```python
from build123d import *

# Parameters (mm, degrees)
F0_R      = 7.5
F1_DEPTH  = 5
F1_FACE_R = 7.5
F2_DEPTH  = 10
F2_TAPER  = 20


with BuildPart() as f1:
    # F0 (on Top) → F1 (new body)
    with BuildSketch(Plane.XY):
        Circle(F0_R)
    extrude(amount=F1_DEPTH)

    # F1_face (on face) → F2 (join)
    with BuildSketch(Plane.XY.offset(5)):
        Circle(F1_FACE_R)
    extrude(amount=F2_DEPTH, taper=F2_TAPER)

    # F3 (on Front) → F4 (revolve)
    with BuildSketch(Plane.XZ):
        with BuildLine():
            Line((0, 23), (0, 10))
            ThreePointArc((0, 10), (6.5, 16.5), (0, 23))
        make_face()
    revolve(axis=Axis((0, 0, 16.5), (0, 0, 1)))


solid = f1.part
```
Can you work these out from the model? Positions are in its coordinate system, mm. Give positions to 0.01 mm unless a question says otherwise; leave off trailing zeros. Loops run counter-clockwise (first coordinate to the right, second up) from the corner with the lowest first, then second, coordinate; pieces in that order, holes last. Notation, with made-up numbers: M 49.5,69 L 88.5,69 A15 cw 88.5,89 Z; hole C 7,52 d4. An arc over 180 degrees is marked long. One line per question, with ' | ' between items. Start each with the question number.
Q1. If we mould it in two halves opening along Z, with no side actions, what happens to faces 1 (the conical face through (5.33, 1.68, 10.25)), 2 (the cylindrical face through (-7.493, 0.33, 2.465)), 3 (the flat face through (0, 0, 0))? For each: +Z half, -Z half, draft (parallel to the pull), parting line (faces both ways), or undercut.
Q2. If we section it at A-A (x = 0): Please give me the cut outline in (y, z).
Q3. If we section it at C-C (z = 17.5): Please give me the cut outline in (x, y).
Q4. For pin 1 Ø6 at (y, z) = (-3, 14) entering from +X; pin 2 Ø1.5 at (y, z) = (-1, 9) entering from +X; pin 3 Ø1 at (x, z) = (-0.5, 18) entering from +Y, each with a flat end and sliding along its axis, tell me the tip position at first contact or that it passes through.
Q5. If I drill on line 1 (X direction, y = 1.5, z = 10.5); line 2 (X direction, y = -3, z = 20.5); line 3 (Y direction, x = -0.5, z = 2), over which ranges is the centre line in solid material (lowest first)? Write a range as from..to.
Q6. If we section it at D-D (z = 7): Please give me the cut outline in (x, y).
Computed:
1) face 1: undercut | face 2: draft | face 3: -Z half
2) outline: M -7.5,0 L 7.5,0 L 7.5,5 L 4.88,12.2 A6.5 ccw long -4.88,12.2 L -7.5,5 Z
3) outline: C 0,0 d12.85
4) pin 1: stops at x = 6.44 | pin 2: stops at x = 6.26 | pin 3: stops at y = 6.41
5) line 1: x = -5.29..5.29 | line 2: x = -4.15..4.15 | line 3: y = -7.48..7.48
6) outline: C 0,0 d13.54
